Geometry check sheet. Reference: the model listing, model coordinates, mm. A direction names the side the tool comes from. Give positions to 0.01 mm unless a question says otherwise; leave off trailing zeros. Order: outer loops, then holes, each group sorted by start corner. A loop starts at its lowest first (then second) coordinate and runs counter-clockwise, first axis right, second up. Notation, with made-up numbers: M 16,73 L 42,73 A17 cw 42,93 Z; hole C -10,79.5 d11. An arc over 180 degrees is marked long. Answer as a JSON object with one key per item and string values. Group by question number.
from build123d import *

# Parameters (mm, degrees)
SKETCH1_W           = 30
SKETCH1_H           = 27.727272728
BOSS_EXTRUDE1_DEPTH = 2
SKETCH2_W           = 10.248894408
SKETCH2_H           = 19.156033471
CUT_EXTRUDE1_DEPTH  = 2
FILLET1_R           = 0.5
FILLET2_R           = 0.5
FILLET3_R           = 0.5
FILLET4_R           = 0.5
FILLET5_R           = 0.5


with BuildPart() as part:
    # Sketch1 → Boss-Extrude1 (new body)
    with BuildSketch(Plane.XY):
        Rectangle(SKETCH1_W, SKETCH1_H)
    extrude(amount=BOSS_EXTRUDE1_DEPTH)

    # Sketch2 → Cut-Extrude1 (cut)
    with BuildSketch(Plane.XY.offset(2)):
        with Locations((0, -4.294276099)):
            Rectangle(SKETCH2_W, SKETCH2_H)
    extrude(amount=-CUT_EXTRUDE1_DEPTH, mode=Mode.SUBTRACT)

    # Fillet1
    fillet1_edges = [part.edges().sort_by_distance(p)[0] for p in [
        (-15, 0, 2),
    ]]
    fillet(fillet1_edges, radius=FILLET1_R)

    # Fillet2
    fillet2_edges = [part.edges().sort_by_distance(p)[0] for p in [
        (15, 0, 2),
    ]]
    fillet(fillet2_edges, radius=FILLET2_R)

    # Fillet3
    fillet3_edges = [part.edges().sort_by_distance(p)[0] for p in [
        (-5.124447204, -4.289947863, 2),
    ]]
    fillet(fillet3_edges, radius=FILLET3_R)

    # Fillet4
    fillet4_edges = [part.edges().sort_by_distance(p)[0] for p in [
        (5.124447204, -4.289947863, 2),
    ]]
    fillet(fillet4_edges, radius=FILLET4_R)

    # Fillet5
    fillet5_edges = [part.edges().sort_by_distance(p)[0] for p in [
        (0, 5.283740637, 2),
    ]]
    fillet(fillet5_edges, radius=FILLET5_R)


solid = part.part
1. Thickness scan on line 1 along X through (y, z) = (-4.5, 1.2); line 2 along Y through (x, z) = (3.75, 1.25); line 3 along X through (y, z) = (-0.25, 1.7). Record the ranges inside material, lowest first. Write a range as [from, to].
2. Access from +Z, -Z, +X, -X, +Y, -Y to the whole of each face (thin tool, end or side, straight path). Record for faces 4 (the flat face through (0, 5.284, 1)), 5 (the flat face through (0, 6, 0)).
3. Depth check by flat-ended pin: pin 1 (1.2 mm diameter, centred on x = 1.5, z = 1, fed in from -Y); pin 2 (2 mm diameter, centred on x = -4.5, y = -3, fed in from +Z). Enter the tip coordinate at first touch or a pass-through.
4. Cross-section at C-C (x = -2.75). Record the cut outline in (y, z), and give its area (3 significant figures).
5. Cross-section at B-B (z = 1.15). Record the cut outline in (x, y).
6. Cross-section at A-A (y = 1.75). Record the cut outline in (x, z).
7. Release check for a two-part mould opening along X. For faces 1 (the flat face through (-10, -13.864, 1)), 2 (the flat face through (15, 0, 1)), 3 (the flat face through (-5.124, -4, 1)) record: released by +X, released by -X, zero draft, split by the parting line, or undercut.
Report:
{
 "1": {"line 1": "x = [-15, -5.12], [5.12, 15]", "line 2": "y = [5.28, 13.86]", "line 3": "x = [-14.96, -5.17], [5.17, 14.96]"},
 "2": {"face 4": "+Z, -Z, -Y", "face 5": "-Z, +X, -X, +Y, -Y"},
 "3": {"pin 1": "stops at y = 5.28", "pin 2": "stops at z = 1.98"},
 "4": {"outline": "M 5.28,0 L 13.86,0 L 13.86,2 L 5.78,2 A0.5 ccw 5.28,1.5 Z", "area": "17.1 mm2"},
 "5": {"outline": "M -15,-13.86 L -5.12,-13.86 L -5.12,5.28 L 5.12,5.28 L 5.12,-13.86 L 15,-13.86 L 15,13.86 L -15,13.86 Z"},
 "6": {"outline": "M -15,0 L -5.12,0 L -5.12,1.5 A0.5 ccw -5.62,2 L -14.5,2 A0.5 ccw -15,1.5 Z; M 5.12,0 L 15,0 L 15,1.5 A0.5 ccw 14.5,2 L 5.62,2 A0.5 ccw 5.12,1.5 Z"},
 "7": {"face 1": "zero draft", "face 2": "released by +X", "face 3": "undercut"}
}
